Design review of the part built by this model. Coordinates are the model's own, in mm. A direction names the side the tool comes from. Round coordinates to 2 decimals unless told otherwise and drop trailing zeros. Write each loop counter-clockwise with the first axis right and the second up, starting at its lowest first coordinate (ties: lowest second). Pieces come first, ordered by that corner, then holes. Notation, with made-up numbers: (-33.75, 65) -> (14.25, 65) arc R13 cw to (14.25, 81) -> close; hole circle Ø3 at (31.5, -27.5). An arc over 180 degrees is marked (long way). One line per question, with ' | ' between items. Start each with the question number.
1) Mouldability with a two-part tool opening along X and no side actions: class faces 5 (the flat face through (-490.59, -113, -10)), 6 (the flat face through (99, 127, 30.755)), 7 (the flat face through (-340.839, -1.883, -9.805)), 8 (the flat face through (-510.3, -112, -21.6)) as +X half, -X half, draft (parallel to the pull), parting line (faces both ways), or undercut.
2) Consider section B-B (x = -602). Give the boundary of the cut face in (y, z).
3) Consider section A-A (y = -168). Give the boundary of the cut face in (x, z).
4) For probe 1 along X at (y, z) = (-54, 12); probe 2 along Y at (x, z) = (-635, -32.5); probe 3 along Z at (x, y) = (866.5, 57.5), list the stretches that pass through material, from the lowest coordinate up.
5) Consider section C-C (z = -73). Give the boundary of the cut face in (x, y), then the cut area to 3 significant figures.
6) For faces 1 (the flat face through (-609, -28.288, -10)), 2 (the flat face through (522.45, 123.48, -9.8)), 3 (the flat face through (912, 35, -57.245)), 4 (the flat face through (-238, 3, 6.755)), list the 3-axis set-ups (+Z, -Z, +X, -X, +Y, -Y) from which the entire face can be reached by the end or side of a thin tool; tool diameter is ignored.
7) Insertion check: pin 1 Ø12 at (x, y) = (-508.5, -112) entering from -Z; pin 2 Ø24 at (y, z) = (-119, -2.5) entering from +X; pin 3 Ø12 at (x, z) = (429, -22.5) entering from +Y. Each pin has a flat end and moves straight along its axis. Give the tip position at first contact, or say it passes through.
```python
from build123d import *

# Parameters (mm, degrees)
SKICA1_R                 = 5.25
P_IDAT_VYSUNUT_M1_DEPTH  = 5
ZAOBLIT1_R               = 4
P_IDAT_VYSUNUT_M3_DEPTH  = 5
SKICA5_R                 = 4.25
SKICA5_R_2               = 1.75
P_IDAT_VYSUNUT_M4_DEPTH  = 1
SKICA8_R                 = 1.05
ODEBRAT_VYSUNUT_M3_DEPTH = 6
ODEBRAT_VYSUNUT_M4_DEPTH = 7
ODEBRAT_START            = -10
SKICA2_R                 = 1.75
ODEBRAT_VYSUNUT_M5_DEPTH = 10
SKICA10_R                = 3.5
ODEBRAT_VYSUNUT_M6_DEPTH = 3
ODEBRAT_START_2          = 50
SKICA11_R                = 0.75
ODEBRAT_VYSUNUT_M7_DEPTH = 10
P_IDAT_VYSUNUT_M5_DEPTH  = 10
P_IDAT_VYSUNUT_M6_DEPTH  = 8
ZAOBLIT2_R               = 2
ODEBRAT_START_3          = -7
ODEBRAT_VYSUNUT_M8_DEPTH = 7
SCALE1_SCALE             = 8


with BuildPart() as part:
    # Skica1 → Přidat vysunutím1 (new, symmetric)
    with BuildSketch(Plane.XY):
        with BuildLine():
            Line((0, 0), (0, 16))
            Line((0, 16), (24, 16))
            Line((24, 16), (24, 0))
            Line((24, 0), (29, 0))
            Line((29, 0), (97.312746067, 39.440382331))
            ThreePointArc((97.312746067, 39.440382331), (105.473420704, 36.802978572), (112.433277726, 41.81425579))
            Line((112.433277726, 41.81425579), (195.687578405, 27.134276321))
            ThreePointArc((195.687578405, 27.134276321), (209.374429572, 27.607666525), (196.674905514, 32.733686604))
            Line((196.674905514, 32.733686604), (113.420604835, 47.413666074))
            ThreePointArc((113.420604835, 47.413666074), (102.174688824, 55.511016714), (94.812746067, 43.77050935))
            Line((94.812746067, 43.77050935), (29, 5.773502692))
            Line((29, 5.773502692), (29, 21))
            Line((29, 21), (-5, 21))
            Line((-5, 21), (-5, 0))
            Line((-5, 0), (0, 0))
        make_face()
        with Locations((104, 46.188021535)):
            Circle(SKICA1_R, mode=Mode.SUBTRACT)
    extrude(amount=P_IDAT_VYSUNUT_M1_DEPTH, both=True)

    # Zaoblit1
    zaoblit1_edges = [part.edges().sort_by_distance(p)[0] for p in [
        (-5, 21, 0),
    ]]
    fillet(zaoblit1_edges, radius=ZAOBLIT1_R)

    # Skica4 → Přidat vysunutím3 (add, symmetric)
    with BuildSketch(Plane.XY):
        Polygon((29, 21), (66.969109888, 27.694978507), (59.37284323, 23.309271907), (29, 17.953720164), align=None)
    extrude(amount=P_IDAT_VYSUNUT_M3_DEPTH, both=True)

    # Skica5 → Přidat vysunutím4 (add)
    with BuildSketch(Plane.XY.offset(5)):
        with Locations((202.480775301, 28.823203768)):
            Circle(SKICA5_R)
        with Locations((202.480775301, 28.823203768)):
            Circle(SKICA5_R_2, mode=Mode.SUBTRACT)
    extrude(amount=P_IDAT_VYSUNUT_M4_DEPTH)

    # Skica8 → Odebrat vysunutím3 (cut)
    with BuildSketch(Plane.XZ):
        with Locations(Location((-1.5, 0, 0), (0, 0, 270))):
            Circle(SKICA8_R)
        with Locations(Location((25.5, 0, 0), (0, 0, 270))):
            Circle(SKICA8_R)
    extrude(amount=-ODEBRAT_VYSUNUT_M3_DEPTH, mode=Mode.SUBTRACT)

    # Skica9 → Odebrat vysunutím4 (cut)
    with BuildSketch(Plane.XY.offset(5)):
        Polygon((24, 16), (29, 16), (29, 13), (24, 8), align=None)
    extrude(amount=-ODEBRAT_VYSUNUT_M4_DEPTH, mode=Mode.SUBTRACT)

    # Skica2 → Odebrat vysunutím5 (cut)
    with BuildSketch(Plane.XY.offset(5).offset(ODEBRAT_START)):
        with Locations((202.480775301, 28.823203768)):
            Circle(SKICA2_R)
    extrude(amount=ODEBRAT_VYSUNUT_M5_DEPTH, mode=Mode.SUBTRACT)

    # Skica10 → Odebrat vysunutím6 (cut)
    with BuildSketch(Plane(origin=(0, 0, -5), x_dir=(-1, 0, 0), z_dir=(0, 0, -1))):
        with Locations((-202.480775301, 28.823203768)):
            Circle(SKICA10_R)
    extrude(amount=-ODEBRAT_VYSUNUT_M6_DEPTH, mode=Mode.SUBTRACT)


with BuildPart() as body_2:
    # Zrcadlit1: mirrored copy
    add(part.part.mirror(Plane(origin=(93.65445241, 28.310869093, -5), x_dir=(1, 0, 0), z_dir=(0, 0, -1))))

    # Skica11 → Odebrat vysunutím7 (cut)
    with BuildSketch(Plane(origin=(0, 0, 0), x_dir=(1, 0, 0), z_dir=(0, 1, 0)).offset(ODEBRAT_START_2)):
        with Locations(Location((103.960302418, 10, 0), (0, 0, 90))):
            Circle(SKICA11_R)
    extrude(amount=ODEBRAT_VYSUNUT_M7_DEPTH, mode=Mode.SUBTRACT)

    # Skica12 → Přidat vysunutím5 (add)
    with BuildSketch(Plane(origin=(0, 0, -15), x_dir=(-1, 0, 0), z_dir=(0, 0, -1))):
        with BuildLine():
            Line((-209.480775301, 28.823203768), (-209.480775301, 16.823203768))
            Line((-209.480775301, 16.823203768), (-195.687578405, 16.823203768))
            Line((-195.687578405, 16.823203768), (-195.687578405, 27.134276321))
            ThreePointArc((-195.687578405, 27.134276321), (-203.331546047, 21.875096894), (-209.480775301, 28.823203768))
        make_face()
    extrude(amount=-P_IDAT_VYSUNUT_M5_DEPTH)

    # Skica13 → Přidat vysunutím6 (add)
    with BuildSketch(Plane(origin=(0, 0, -15), x_dir=(-1, 0, 0), z_dir=(0, 0, -1))):
        Polygon((-204.334176853, 20.823203768), (-200.834176853, 20.823203768), (-198.334176853, 16.823203768), (-206.834176853, 16.823203768), align=None)
    extrude(amount=P_IDAT_VYSUNUT_M6_DEPTH)

    # Zaoblit2
    zaoblit2_edges = [body_2.edges().sort_by_distance(p)[0] for p in [
        (195.687578405, 16.823203768, -10),
        (209.480775301, 16.823203768, -10),
    ]]
    fillet(zaoblit2_edges, radius=ZAOBLIT2_R)

    # Skica14 → Odebrat vysunutím8 (cut)
    with BuildSketch(Plane(origin=(0, 0, -15), x_dir=(-1, 0, 0), z_dir=(0, 0, -1)).offset(ODEBRAT_START_3)):
        Polygon((-59.37284323, 23.309271907), (-66.969109888, 27.694978507), (-61.786216453, 26.781094556), (-54.189949795, 22.395387956), align=None)
    extrude(amount=ODEBRAT_VYSUNUT_M8_DEPTH, mode=Mode.SUBTRACT)


with BuildPart() as body_2_1:
    # Scale1: scaled about (103.22707652, 28.04115128, -10.107869414)
    add(body_2.part.scale(SCALE1_SCALE).moved(Location((-722.58953564, -196.28805896, 70.755085898))))


solid = body_2_1.part
```
From the geometry:
1) face 5: undercut | face 6: draft | face 7: -X half | face 8: undercut
2) outline: (-68.29, -49.24) -> (-28.29, -49.24) -> (-28.29, 30.76) -> (-68.29, 30.76) -> close
3) outline: (-762.59, -49.24) -> (-722.59, -49.24) -> (-722.59, 30.76) -> (-762.59, 30.76) -> close; (-530.59, -49.24) -> (-441.59, -49.24) -> (-441.59, 30.76) -> (-530.59, 30.76) -> close; hole circle Ø16.8 at (-734.59, -9.24); hole circle Ø16.8 at (-518.59, -9.24)
4) probe 1: x = -761.97 to -490.59, -324.14 to -244.14, 845.23 to 950.94 | probe 2: y = -68.29 to -28.29 | probe 3: z = -49.24 to 30.76
5) outline: (864.08, -61.7) -> (932.08, -61.7) -> (912.08, -29.7) -> (884.08, -29.7) -> close | area: 1,540 mm2
6) face 1: +Z, -Z, -X, +Y | face 2: +Z, -Z, +Y | face 3: -Z, +X, -X, +Y | face 4: -Z
7) pin 1: stops at z = -49.24 | pin 2: stops at x = -335.94 | pin 3: stops at y = 141.02
